```python
from build123d import *

# Parameters (mm, degrees)
BOSS_EXTRUDE1_DEPTH = 9
SKETCH4_W           = 31
SKETCH4_H           = 8
SKETCH4_H_2         = 6
BOSS_EXTRUDE4_DEPTH = 45
CUT_EXTRUDE1_DEPTH  = 58
SKETCH6_3_R         = 11.25
CUT_EXTRUDE2_DEPTH  = 6
CUT_EXTRUDE3_DEPTH  = 4.3
CUT_EXTRUDE4_DEPTH  = 2.2
SKETCH9_3_R         = 4.65
CUT_EXTRUDE5_DEPTH  = 8
SKETCH13_W          = 14
SKETCH13_H          = 5
CUT_EXTRUDE8_DEPTH  = 9
SKETCH14_R          = 1.75
CUT_EXTRUDE9_DEPTH  = 3


with BuildPart() as part:
    # Sketch1 → Boss-Extrude1 (new body)
    with BuildSketch(Plane.XY):
        Polygon((15.5, -28.5), (-15.5, -28.5), (-15.5, -10.3), (-15.5, 10.3), (-15.5, 28.5), (15.5, 28.5), align=None)
    extrude(amount=BOSS_EXTRUDE1_DEPTH)

    # Sketch4 → Boss-Extrude4 (add)
    with BuildSketch(Plane(origin=(0, 0, 0), x_dir=(-1, 0, 0), z_dir=(0, 0, -1))):
        with Locations((0, 24.5)):
            Rectangle(SKETCH4_W, SKETCH4_H)
        with Locations((0, -25.5)):
            Rectangle(SKETCH4_W, SKETCH4_H_2)
    extrude(amount=BOSS_EXTRUDE4_DEPTH)

    # Sketch6 → Cut-Extrude1 (cut, through all)
    with BuildSketch(Plane.XZ.offset(28.5)):
        with BuildLine():
            ThreePointArc((15.5, -29.5), (10.960155101, -40.460155116), (-2.1e-08, -45))
            Line((-2.1e-08, -45), (15.5, -45))
            Line((15.5, -45), (15.5, -29.5))
        make_face()
        with BuildLine():
            ThreePointArc((-2.1e-08, -45), (-10.960155116, -40.460155101), (-15.5, -29.5))
            Line((-15.5, -29.5), (-15.5, -45))
            Line((-15.5, -45), (-2.1e-08, -45))
        make_face()
    extrude(amount=-CUT_EXTRUDE1_DEPTH, mode=Mode.SUBTRACT)

    # Sketch6<3> → Cut-Extrude2 (cut)
    with BuildSketch(Plane.XZ.offset(28.5)):
        with Locations((0, -29.5)):
            Circle(SKETCH6_3_R)
    extrude(amount=-CUT_EXTRUDE2_DEPTH, mode=Mode.SUBTRACT)

    # Sketch7 → Cut-Extrude3 (cut)
    with BuildSketch(Plane(origin=(0, 28.5, 0), x_dir=(1, 0, 0), z_dir=(0, 1, 0))):
        with BuildLine():
            Line((-17.1, 31.65), (-4.313351365, 33.813351365))
            Line((-4.313351365, 33.813351365), (-2.15, 46.6))
            ThreePointArc((-2.15, 46.6), (0, 48.75), (2.15, 46.6))
            Line((2.15, 46.6), (4.313351365, 33.813351365))
            Line((4.313351365, 33.813351365), (17.1, 31.65))
            ThreePointArc((17.1, 31.65), (19.25, 29.5), (17.1, 27.35))
            Line((17.1, 27.35), (4.313351365, 25.186648635))
            Line((4.313351365, 25.186648635), (2.15, 12.4))
            ThreePointArc((2.15, 12.4), (0, 10.25), (-2.15, 12.4))
            Line((-2.15, 12.4), (-4.313351365, 25.186648635))
            Line((-4.313351365, 25.186648635), (-17.1, 27.35))
            ThreePointArc((-17.1, 27.35), (-19.25, 29.5), (-17.1, 31.65))
        make_face()
    extrude(amount=-CUT_EXTRUDE3_DEPTH, mode=Mode.SUBTRACT)

    # Sketch9 → Cut-Extrude4 (cut)
    with BuildSketch(Plane.XZ.offset(-20.5)):
        with BuildLine():
            ThreePointArc((3.25, -32.82565783), (0, -34.15), (-3.25, -32.82565783))
            Line((-3.25, -32.82565783), (-3.25, -44.655444566))
            ThreePointArc((-3.25, -44.655444566), (0, -45), (3.25, -44.655444566))
            Line((3.25, -44.655444566), (3.25, -32.82565783))
        make_face()
    extrude(amount=-CUT_EXTRUDE4_DEPTH, mode=Mode.SUBTRACT)

    # Sketch9<3> → Cut-Extrude5 (cut)
    with BuildSketch(Plane.XZ.offset(-20.5)):
        with Locations((0, -29.5)):
            Circle(SKETCH9_3_R)
    extrude(amount=-CUT_EXTRUDE5_DEPTH, mode=Mode.SUBTRACT)

    # Sketch13 → Cut-Extrude8 (cut)
    with BuildSketch(Plane(origin=(0, 28.5, 0), x_dir=(1, 0, 0), z_dir=(0, 1, 0))):
        with Locations((0, 3.5)):
            Rectangle(SKETCH13_W, SKETCH13_H)
    extrude(amount=-CUT_EXTRUDE8_DEPTH, mode=Mode.SUBTRACT)

    # Sketch14 → Cut-Extrude9 (cut)
    with BuildSketch(Plane.XY.offset(9)):
        with Locations((11.31642939, 25)):
            Circle(SKETCH14_R)
        with Locations((-11.31642939, 25)):
            Circle(SKETCH14_R)
        with Locations((11.31642939, -25)):
            Circle(SKETCH14_R)
        with Locations((-11.31642939, -25)):
            Circle(SKETCH14_R)
    extrude(amount=-CUT_EXTRUDE9_DEPTH, mode=Mode.SUBTRACT)


solid = part.part
```
Work out the finished part from the listing and answer in its coordinate system (mm). A direction names the side the tool comes from. Give positions to 0.01 mm unless a question says otherwise; leave off trailing zeros. Write each loop counter-clockwise with the first axis right and the second up, starting at its lowest first coordinate (ties: lowest second). Pieces come first, ordered by that corner, then holes.
(1) Which of the six approach directions +Z, -Z, +X, -X, +Y, -Y give full straight-line access (tool end or side, diameter ignored) to faces 5 (the cylindrical face through (5.19, -25.54, -39.48)), 6 (the flat face through (0, 20.5, -22)), 7 (the flat face through (-7, 25, -3)), 8 (the flat face through (0, 0, 9)), 9 (the flat face through (11, -25, 6))?
Final values:
face 5: -Y
face 6: -Z, +X, -X
face 7: +Y
face 8: +Z, +X, -X, +Y, -Y
face 9: +Z
(2) Straight lines are drawn through the part: line 1 (Y direction, x = -12.5, z = -37); line 2 (Y direction, x = -2, z = -14); line 3 (Y direction, x = 2, z = -25). For each, find the intervals that lie inside material, in ascending order.
Final values:
line 1: y = -28.5 to -22.5, 20.5 to 28.5
line 2: y = -28.5 to -22.5, 20.5 to 24.2
line 3: y = 20.5 to 24.2
(3) The part is cut by section B-B on z = -8. Write down the section's boundary in (x, y).
Final values:
outline: (-15.5, -28.5) - (15.5, -28.5) - (15.5, -22.5) - (-15.5, -22.5) - close; (-15.5, 20.5) - (15.5, 20.5) - (15.5, 28.5) - (-15.5, 28.5) - close
(4) The mould has two halves that part along Y. Classify faces 1 (the flat face through (-11, -25, 6)), 2 (the flat face through (9, 28.5, -38)), 3 (the cylindrical face through (11.089, 26.735, 7.521)), 4 (the flat face through (-9.89, 26.38, -32.87)): pulls with the +Y half, pulls with the -Y half, needs draft (parallel to the pull), parting line crosses it, or undercut.
Final values:
face 1: undercut
face 2: pulls with the +Y half
face 3: undercut
face 4: needs draft
(5) The part is cut by section C-C on z = -20. Write down the section's boundary in (x, y), plus the area to 3 significant figures.
Final values:
outline: (-15.5, -28.5) - (-6.03, -28.5) - (-6.03, -22.5) - (-15.5, -22.5) - close; (-15.5, 20.5) - (15.5, 20.5) - (15.5, 28.5) - (3.44, 28.5) - (3.44, 24.2) - (-3.44, 24.2) - (-3.44, 28.5) - (-15.5, 28.5) - close; (6.03, -28.5) - (15.5, -28.5) - (15.5, -22.5) - (6.03, -22.5) - close
area: 332 mm2
(6) The part is cut by section D-D on x = -5.5. Write down the section's boundary in (y, z), plus the area to 3 significant figures.
Final values:
outline: (-28.5, -43.99) - (-22.5, -43.99) - (-22.5, -39.31) - (-28.5, -39.31) - close; (-28.5, -19.69) - (-22.5, -19.69) - (-22.5, 0) - (20.5, 0) - (20.5, -1) - (28.5, -1) - (28.5, 9) - (-28.5, 9) - close; (20.5, -43.99) - (28.5, -43.99) - (28.5, -33.61) - (24.2, -33.61) - (24.2, -25.39) - (28.5, -25.39) - (28.5, -6) - (20.5, -6) - close
area: 936 mm2
(7) Flat-ended cylindrical pins translate along their axes: pin 1 Ø1 at (x, y) = (7.5, -15.5) entering from -Z; pin 2 Ø13.5 at (x, z) = (0, -29.5) entering from -Y; pin 3 Ø1.8 at (x, y) = (-11.5, -25) entering from +Z. Find the tip coordinate at first contact, or state that the pin passes through.
Final values:
pin 1: stops at z = 0
pin 2: stops at y = 20.5
pin 3: stops at z = 6
(8) The part is cut by section A-A on y = 25. Write down the section's boundary in (x, z), plus the area to 3 significant figures.
Final values:
outline: (-15.5, -27.08) - (-4.31, -25.19) - (-2.15, -12.4) arc R2.15 cw to (2.15, -12.4) - (4.31, -25.19) - (15.5, -27.08) - (15.5, 9) - (13.07, 9) - (13.07, 6) - (9.57, 6) - (9.57, 9) - (-9.57, 9) - (-9.57, 6) - (-13.07, 6) - (-13.07, 9) - (-15.5, 9) - close; (-15.3, -31.95) arc R15.5 ccw to (-2.45, -44.8) - (-4.31, -33.81) - close; (2.45, -44.8) arc R15.5 ccw to (15.3, -31.95) - (4.31, -33.81) - close; hole (-7, -6) - (7, -6) - (7, -1) - (-7, -1) - close
area: 1,090 mm2
